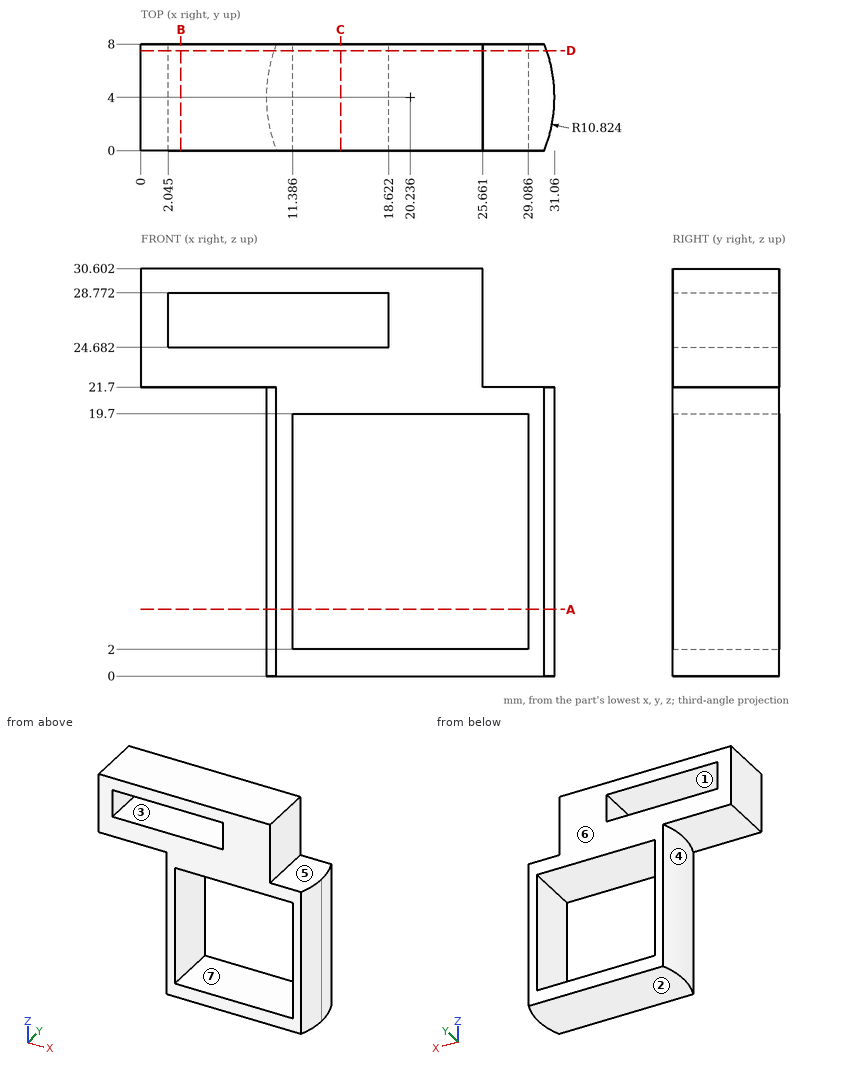
Geometry: see drawing. Coordinates: mm, zero at the bounding-box minimum. A direction names the side the tool comes from. Coordinates: 2 decimals unless noted, no trailing zeros. Loops run counter-clockwise (first coordinate to the right, second up) from the corner with the lowest first, then second, coordinate; pieces in that order, holes last. Notation, with made-up numbers: M -9.75,82 L 31.25,82 A12 cw 31.25,92 Z; hole C 88,-30.75 d5. An arc over 180 degrees is marked long. Put each result on its own line as item: value. Start each with the question number.
1) Cut plane C-C on x = 15. Return the cut outline in (y, z).
2) Contact query for flat-ended pins moving along their axis: pin 1 Ø1.5 at (x, z) = (13.5, 9.5) entering from +Y; pin 2 Ø4.5 at (y, z) = (3.5, 26) entering from +X. Output: stop coordinate, or through.
3) Reachability of the marked faces 5, 6 and 7 from +Z, -Z, +X, -X, +Y, -Y: full face, straight path, thin tool, end or side. Return the list, or none.
4) Cut plane B-B on x = 3. Return the cut outline in (y, z), then the cut area to 3 significant figures.
5) Cut plane A-A on z = 5. Return the cut outline in (x, y).
6) Pull-direction query (Z, two-part tool) for the marked faces 1, 2, 3 and 4; classes: pulls with the +Z half, pulls with the -Z half, needs draft (parallel to the pull), parting line crosses it, or undercut.
7) Cut plane D-D on y = 7.5. Return the cut outline in (x, z) (1 decimal).
8) Ray query, L1, parallel to Z at x = 16, y = 6.5; L2, parallel to Z at x = 20, y = 3.75; L3, parallel to Z at x = 5, y = 3.25. Return the intervals inside material, ascending. Write a range as from..to.
The answers:
1. outline: M 0,0 L 8,0 L 8,2 L 0,2 Z; M 0,19.7 L 8,19.7 L 8,24.68 L 0,24.68 Z; M 0,28.77 L 8,28.77 L 8,30.6 L 0,30.6 Z
2. pin 1: passes through
2. pin 2: stops at x = 25.66
3. face 5: +Z, +X, +Y, -Y
3. face 6: +Z, -Z, +X, -X, +Y
3. face 7: +Y, -Y
4. outline: M 0,21.7 L 8,21.7 L 8,24.68 L 0,24.68 Z; M 0,28.77 L 8,28.77 L 8,30.6 L 0,30.6 Z
4. area: 38.5 mm²
5. outline: M 10.18,0 L 11.39,0 L 11.39,8 L 10.18,8 A10.82 ccw Z; M 29.09,0 L 30.29,0 A10.82 ccw 30.29,8 L 29.09,8 Z
6. face 1: undercut
6. face 2: pulls with the -Z half
6. face 3: undercut
6. face 4: needs draft
7. outline: M 0,21.7 L 10,21.7 L 10,0 L 30.5,0 L 30.5,21.7 L 25.7,21.7 L 25.7,30.6 L 0,30.6 Z; hole M 2,24.7 L 18.6,24.7 L 18.6,28.8 L 2,28.8 Z; hole M 11.4,2 L 29.1,2 L 29.1,19.7 L 11.4,19.7 Z
8. L1: z = 0..2, 19.7..24.68, 28.77..30.6
8. L2: z = 0..2, 19.7..30.6
8. L3: z = 21.7..24.68, 28.77..30.6
